from build123d import *

# Parameters (mm, degrees)
F4_R      = 22
F4_R_2    = 4.025
F5_DEPTH  = 1.6
F6_DEPTH  = 7
F8_SIZE   = 1
F9_DEPTH  = 20
F10_COUNT = 11
F11_START = 21.6
F11_DEPTH = 1.6


with BuildPart() as f5:
    # F4 (on Top) → F5 (new body)
    with BuildSketch(Plane.XY):
        Circle(F4_R)
        Circle(F4_R_2, mode=Mode.SUBTRACT)
        Circle(F4_R_2)
    extrude(amount=F5_DEPTH)

    # F4 (on Top) → F6 (join)
    with BuildSketch(Plane.XY):
        Circle(F4_R_2)
    extrude(amount=-F6_DEPTH)

    # F8
    f8_edges = [f5.edges().sort_by_distance(p)[0] for p in [
        (-4.025, 0, -7),
    ]]
    chamfer(f8_edges, length=F8_SIZE)



with BuildPart() as f9:
    # F7 (on face) → F9 (new body)
    with BuildSketch(Plane.XY.offset(1.6)):
        with BuildLine():
            ThreePointArc((0, -1.6), (0.8, -0.8), (0, 0))
            ThreePointArc((0, 0), (-11, -11), (0, -22))
            ThreePointArc((0, -22), (0.8, -21.2), (0, -20.4))
            ThreePointArc((0, -20.4), (-9.4, -11), (0, -1.6))
        make_face()
    extrude(amount=F9_DEPTH)


with BuildPart() as f5_1:
    add(f5.part)

    add(f9.part)  # F10 merges F9
    # F10: F9 ×11 about axis
    f10_axis = Axis((0, 0, 0), (0, 0, 1))
    for i in range(1, F10_COUNT):
        add(f9.part.rotate(f10_axis, i * 360 / F10_COUNT))

    # F4 (on Top) → F11 (join)
    with BuildSketch(Plane.XY.offset(F11_START)):
        Circle(F4_R)
        Circle(F4_R_2, mode=Mode.SUBTRACT)
        Circle(F4_R_2)
    extrude(amount=F11_DEPTH)


solid = f5_1.part
Input: part model. Units: mm. Frame: model coordinates. A direction names the side the tool comes from. Round coordinates to 2 decimals unless told otherwise and drop trailing zeros. Order: outer loops, then holes, each group sorted by start corner. A loop starts at its lowest first (then second) coordinate and runs counter-clockwise, first axis right, second up.
1. Material intervals for line 1 (Z direction, x = -10, y = 14.5); line 2 (X direction, y = 9, z = 5.5); line 3 (Y direction, x = 13, z = 19), sorted ascending.
The answers:
line 1: z = 0 to 1.6, 21.6 to 23.2
line 2: x = -19 to -16.64, -5.14 to -2.78, 0.91 to 2.54, 6.17 to 7.79, 12.37 to 13.99, 17.54 to 19.17
line 3: y = -15.15 to -13.48, -9.23 to -7.59, -2.75 to -0.94, 5.76 to 15.35
2. Cut plane D-D, the plane y = -21.2. Output: boundary loops of the cut face in (x, z).
The answers:
outline: (-5.88, 0) - (5.88, 0) - (5.88, 1.6) - (0.8, 1.6) - (0.8, 21.6) - (5.88, 21.6) - (5.88, 23.2) - (-5.88, 23.2) - (-5.88, 21.6) - (-4.12, 21.6) - (-4.12, 1.6) - (-5.88, 1.6) - close
3. Set-up query: faces 3 (the face through (0.8, -21.2, 11.5)), 4 (the face through (-4.769, -21.477, 0.789)), 5 (the face through (14, 6, 21.6)). Return all of +Z, -Z, +X, -X, +Y, -Y with unobstructed straight access to the full face (end or side cutting, diameter ignored); none if empty.
The answers:
face 3: +X
face 4: +Z, -Z
face 5: none
4. Mould query, pull axis Z, two halves, no side actions, for faces 1 (the face through (0, 0, -7)), 2 (the face through (-2.59, -16.19, 11.46)). Classes: released by +Z, released by -Z, zero draft, split by the parting line, or undercut.
The answers:
face 1: released by -Z
face 2: undercut
5. Pin query (flat end, axial travel): P1, Ø12, axis at x = 12.5, y = 12, coming from the -Z side; P2, Ø12, axis at x = -1, z = -3, coming from the -Y side; P3, Ø3, axis at y = 15, z = 12.5, coming from the -X side; P4, Ø8, axis at y = -13, z = 2.5, coming from the -X side. Return the tip coordinate at first contact, or that it passes through.
The answers:
P1: stops at z = 0
P2: stops at y = -22
P3: stops at x = -16.82
P4: stops at x = -20.07
6. Cut plane A-A, the plane x = 10. State how many separate pieces and enclosed holes the cut face has, then the cut area to 3 significant figures.
The answers:
separate pieces: 1
enclosed holes: 5
area: 344 mm2
